Autodesk Inventor part; units mm, degrees
ref_plane "YZ Plane" through (0, 0, 0) normal (1, 0, 0) x (0, 1, 0)
ref_plane "XY Plane" through (0, 0, 0) normal (0, 0, 1) x (1, 0, 0)
sketch "Sketch1" plane through (0, 0, 0) normal (0, 1, 0) x (-1, 0, 0)
  arc A0 (0, -5) -> (0, 5) centre (0, 0) ccw
  line L0 (0, 5) -> (0, -5)
  dimension "d0" = 10
extrude "Extrusion1" add sketch "Sketch1" along normal blind 10
sketch "Sketch2" plane through (0, 0, 0) normal (1, 0, 0) x (0, 1, 0)
  line L0 (8.0172, -4.5) -> (8.0172, 4.5)
  line L1 (8.0172, 4.5) -> (2.5172, 4.5)
  line L2 (2.5172, -4.5) -> (0.0172, -2)
  line L3 (2.5172, 4.5) -> (0.0172, 2)
  line L4 (0.0172, -2) -> (0.0172, 2)
  line L5 (8.0172, -4.5) -> (2.5172, -4.5)
  point P0 (0, 0)
  dimension "d3" = 9
  dimension "d4" = 8
sketch "Sketch3" plane through (0, 0, 0) normal (1, 0, 0) x (0, 1, 0)
  line L0 (0, 2) -> (3, 5)
  arc A0 (3, 5) -> (0, 2) centre (1, 4) ccw
  line L1 (0, -2) -> (4, -6)
  arc A1 (0, -2) -> (4, -6) centre (1.75, -4.25) ccw
  line L2 (8.0325, 5) -> (11, 5)
  line L3 (11, 5) -> (11, -6)
  line L4 (11, -6) -> (8.0325, -6)
  line L5 (8.0325, -6) -> (8.0325, 5)
  line L6 (2.4911, 4.4911) -> (5, 7)
  line L7 (2.4911, 4.4911) -> (8.0325, 4.4911)
  arc A2 (8.0325, 4.4911) -> (5, 7) centre (7, 6.3303) ccw
  line L8 (2.4911, -4.4911) -> (8.5706, -4.4911)
  arc A3 (2.4911, -4.4911) -> (8.5706, -4.4911) centre (5.5309, -7.5041) ccw
  point P0 (0, 0)
extrude "Extrusion2" cut sketch "Sketch3" against normal through all
sketch "Sketch4" plane through (0, 0, 0) normal (0, 1, 0) x (-1, 0, 0)
  arc A0 (1.0726, -4.4911) -> (1.0726, 4.4911) centre (-1.125, 0) ccw
  arc A1 (1.0726, 4.4911) -> (1.0726, -4.4911) centre (-0.4517, 0) ccw
  point P0 (0, 0)
  point P1 (2.1976, -4.4911)
  point P2 (2.1976, 4.4911)
  dimension "d9" = 1.125
  dimension "d10" = 1.125
extrude "Extrusion3" cut sketch "Sketch4" along normal through all both and the other way through all
sketch "Sketch5" plane through (0, 0, 0) normal (1, 0, 0) x (0, 1, 0)
  line L0 (1.6, -1.2445) -> (1.6, 1.1555)
  line L1 (6.4325, 2.6911) -> (3.1125, 2.6911)
  line L2 (6.4325, -2.6911) -> (6.4325, 2.6911)
  line L3 (6.4325, -2.6911) -> (3.1125, -2.6911)
  line L4 (0, 2) -> (0, -2)
  line L5 (8.0325, 4.4911) -> (8.0325, -4.4911)
  line L6 (0, 2) -> (2.4911, 4.4911)
  line L7 (2.4911, 4.4911) -> (8.0325, 4.4911)
  line L8 (8.0325, 4.4911) -> (8.0325, -4.4911)
  line L9 (8.0325, -4.4911) -> (2.4911, -4.4911)
  line L10 (2.4911, -4.4911) -> (0, -2)
  line L11 (0, 2) -> (0, -2)
  line L12 (1.6, 1.1555) -> (3.1125, 2.6911)
  line L13 (1.6, -1.2445) -> (3.1125, -2.6911)
  line L14 (1.6, 4.6579) -> (1.6, -5.3823)
  arc A0 (1.6, 4.6579) -> (1.6, -5.3823) centre (3.2437, -0.3622) ccw
  line L15 (1.6, 1.1555) -> (5.4757, 5.0906)
  line L16 (1.6, 1.1555) -> (1.6, 7.5999)
  arc A1 (5.4757, 5.0906) -> (1.6, 7.5999) centre (3.8837, 6.8794) ccw
  line L17 (3.1125, 2.6911) -> (12.4034, 2.6911)
  line L18 (3.1125, 2.6911) -> (8.5318, 8.1936)
  arc A2 (12.4034, 2.6911) -> (8.5318, 8.1936) centre (8.3272, 3.9364) ccw
  line L19 (6.4325, 2.6911) -> (13.6333, 2.6911)
  line L20 (6.4325, 2.6911) -> (6.4325, -9.3636)
  arc A3 (6.4325, -9.3636) -> (13.6333, 2.6911) centre (6.37, -1.1482) ccw
  line L21 (6.4325, -2.6911) -> (6.4325, -11.5775)
  line L22 (6.4325, -2.6911) -> (3.1125, -2.6911)
  line L23 (3.1125, -2.6911) -> (3.2437, -12.8567)
  arc A4 (3.2437, -12.8567) -> (6.4325, -9.3636) centre (5.6123, -11.8169) ccw
  line L24 (1.6, -1.2445) -> (1.6, -8.2222)
  line L25 (1.6, -1.2445) -> (3.1125, -2.6911)
  line L26 (3.1125, -2.6911) -> (3.1946, -9.0574)
  arc A5 (1.6, -8.2222) -> (3.1946, -9.0574) centre (2.6381, -8.1801) ccw
  point P0 (0, 0)
  dimension "d16" = 1.6
  dimension "d18" = 1.6
  dimension "d21" = 1.8
  dimension "d23" = 1.8
  dimension "d24" = 2.4
  dimension "d26" = 3.32
  dimension "d27" = 3.32
extrude "Extrusion4" cut sketch "Sketch5" against normal through all contours L14 L10 L4 L6 L0 | L13 L23 L9 L10 L14 | L14 L6 L7 L15 L12 | L3 L20 L9 L23 | L14 A0 L6 L4 L10 | L10 L9 L23 A5 L24 L14 | L15 L7 L5 L17 L1 | L14 L16 A1 L15 L7 L6 | L2 L17 L5 L9 L20 | L9 L20 A4 L23 | L15 L18 A2 L17 L5 L7 | L9 L5 L17 L19 A3 L20
sketch "Sketch6" plane through (0, 0, 0) normal (1, 0, 0) x (0, 1, 0)
  circle A0 centre (4, 0) radius 2.5
  line L0 (1.6, -1.2445) -> (1.6, 1.1555)
  point P0 (0, 0)
  dimension "d31" = 5
  dimension "d32" = 2.4
extrude "Extrusion5" add sketch "Sketch6" against normal blind 15
sketch "Sketch7" plane through (0, 0, 0) normal (0, 1, 0) x (-1, 0, 0)
  arc A0 (3.089, -2.6911) -> (3.7176, -1.2445) centre (-1.125, 0) ccw
  arc A1 (3.7397, 1.1555) -> (3.089, 2.6911) centre (-1.125, 0) ccw
  arc A2 (3.7176, -1.2445) -> (3.7397, 1.1555) centre (-1.125, 0) ccw
  arc A3 (3.089, 2.6911) -> (3.089, -2.6911) centre (1.3425, 0) ccw
  point P0 (0, 0)
extrude "Extrusion6" cut sketch "Sketch7" along normal through all
sketch "Sketch8" plane through (-15, 4, 0) normal (-1, 0, 0) x (0, 0, 1)
  circle A0 centre (0, 0) radius 0.5875
  point P0 (0, -4)
  dimension "d37" = 1.175
extrude "Extrusion7" cut sketch "Sketch8" against normal blind 7
sketch "Sketch9" plane through (0, 0, 0) normal (0, 1, 0) x (-1, 0, 0)
  line L0 (6, 3) -> (2, 3)
  line L1 (2, 3) -> (2, -3)
  line L2 (2, -3) -> (6, -3)
  line L3 (6, -3) -> (6, 3)
  point P0 (0, 0)
extrude "Extrusion8" cut sketch "Sketch9" along normal through all both and the other way through all
sketch "Sketch10" plane through (-15, 4, 0) normal (-1, 0, 0) x (0, 0, 1)
  circle A0 centre (0, 0) radius 1.25
  circle A1 centre (0, 0) radius 3.9528
  point P0 (0, -4)
  dimension "d69" = 2.5
extrude "Extrusion9" cut sketch "Sketch10" against normal blind 8
ref_plane "Work Plane1" through (0, 4.1, 0) normal (0, 1, 0) x (-1, 0, 0)
sketch "Sketch12" plane through (0, 4.1, 0) normal (0, 1, 0) x (-1, 0, 0)
  line L0 (15, -1) -> (15, 1)
  line L1 (5.9113, 12.6879) -> (5.9113, -12.7121)
  line L2 (5.9113, 12.6879) -> (-21.266, 0.1332)
  line L3 (-21.266, 0.1332) -> (5.9113, -12.7121)
  line L4 (7.0341, 14.6962) -> (7.0341, -14.7038)
  line L5 (2.03, -0.0038) -> (19.03, -0.0038)
  line L6 (-25.0887, 5) -> (-25.0887, -5)
  line L7 (-25.0887, 5) -> (7.0341, 14.6962)
  line L8 (-25.0887, -5) -> (7.0341, -14.7038)
  point P0 (0, 0)
  point P1 (0, 0)
  dimension "d61" = 25.4
  dimension "d62" = 29.4
  dimension "d63" = 14.7
  dimension "d64" = 10
  dimension "d67" = 31
extrude "Extrusion11" add sketch "Sketch12" along normal mid plane 2.18
sketch "Sketch13" plane through (25.0887, 3.01, -5) normal (1, 0, 0) x (0, 0, -1)
  circle A0 centre (-5, 0.6559) radius 0.39
  circle A1 centre (-5, 0.6559) radius 0.85
  circle A2 centre (-5, 0.6559) radius 1.09
  point P0 (-5, -3.01)
  dimension "d70" = 0.78
  dimension "d71" = 1.7
  dimension "d74" = 2.18
extrude "Extrusion13" add sketch "Sketch13" along normal blind 30
fillet "Fillet1" radius 2 1 edges at (25.0887, 4.1, -5)
fillet "Fillet2" radius 2 1 edges at (25.0887, 4.1, 5)
properties part number "piezo_mounted_whisk_deflector_SHORT_capillary_attachment"
Work out the finished part from the listing and answer in its coordinate system (mm). A direction names the side the tool comes from. Give positions to 0.01 mm unless a question says otherwise; leave off trailing zeros. Order: outer loops, then holes, each group sorted by start corner. A loop starts at its lowest first (then second) coordinate and runs counter-clockwise, first axis right, second up. Notation, with made-up numbers: (16, -16) -> (50, -16) arc R5 cw to (50, -12) -> close; hole circle Ø10 at (46, -14.5). An arc over 180 degrees is marked (long way). Answer as a JSON object with one key per item and string values. Group by question number.
1. Flat-ended cylindrical pins translate along their axes: pin 1 Ø0.7 at (y, z) = (4, -7) entering from -X; pin 2 Ø0.8 at (y, z) = (2, 1) entering from +X; pin 3 Ø4 at (x, z) = (21.5, -7.5) entering from +Y. Find the tip coordinate at first contact, or state that the pin passes through.
2. Section A-A on x = 9.5 is taken. Determine the outline of the cut face in (y, z), plus the area to 3 significant figures.
3. Consider line 1 along Y through (x, z) = (33, 0); line 2 along X through (y, z) = (2.8, 0.5); line 3 along Y through (x, z) = (-10.5, 0). Determine where each line is inside the solid, lowest interval first. Write a range as [from, to].
4. A tool of negligible diameter and unlimited length cuts with its end or side. For faces 4 (the flat face through (-7, 2, 0)), 5 (the flat face through (-8, 4, 0)), 6 (the flat face through (-5.911, 4, 0)), from which of +Z, -Z, +X, -X, +Y, -Y can it reach the whole face along a straight path? Write none if from no direction.
5. The mould has two halves that part along Y. Classify faces 1 (the cylindrical face through (-11.549, 3.426, -0.127)), 2 (the flat face through (10.3, 5.19, -5.4)), 3 (the flat face through (8.53, 4.08, 10)): released by +Y, released by -Y, zero draft, split by the parting line, or undercut.
6. Section B-B on z = 6.25 is taken. Determine the outline of the cut face in (x, y), plus the area to 3 significant figures.
Result sheet:
{
 "1": {"pin 1": "stops at x = -7.03", "pin 2": "stops at x = -6", "pin 3": "stops at y = 5.19"},
 "2": {"outline": "(3.01, -9.71) -> (5.19, -9.71) -> (5.19, -5.43) -> (3.01, -5.43) -> close; (3.01, 5.57) -> (5.19, 5.57) -> (5.19, 9.71) -> (3.01, 9.71) -> close", "area": "18.4 mm^2"},
 "3": {"line 1": "y = [2.58, 2.82], [3.28, 4.06], [4.52, 4.76]", "line 2": "x = [-7, -6], [25.09, 55.09]", "line 3": "y = [2.75, 3.41], [4.59, 5.25]"},
 "4": {"face 4": "-X, -Y", "face 5": "-X", "face 6": "+Y, -Y"},
 "5": {"face 1": "undercut", "face 2": "released by +Y", "face 3": "zero draft"},
 "6": {"outline": "(-7.03, 3.01) -> (-5.91, 3.01) -> (-5.91, 5.19) -> (-7.03, 5.19) -> close; (8.02, 3.01) -> (20.95, 3.01) -> (20.95, 5.19) -> (8.02, 5.19) -> close", "area": "30.6 mm^2"}
}
